For this review, take the finished solid that the model builds, in its own axes (mm). A direction names the side the tool comes from. Round coordinates to 2 decimals unless told otherwise and drop trailing zeros. Order: outer loops, then holes, each group sorted by start corner. A loop starts at its lowest first (then second) coordinate and runs counter-clockwise, first axis right, second up. Notation, with made-up numbers: (18.5, -3) - (37.5, -3) arc R12 ccw to (37.5, 5) - close; hole circle Ø7 at (1.25, 83). An arc over 180 degrees is marked (long way). One line per item, written item: value.
```python
from build123d import *

# Parameters (mm, degrees)
SKETCH1_W           = 10
SKETCH1_H           = 290
SKETCH2_R           = 15
BOSS_EXTRUDE1_DEPTH = 50


with BuildPart() as part:
    # Sketch1 → Revolve1 (revolve)
    with BuildSketch(Plane.XY, mode=Mode.PRIVATE) as revolve1_sk:
        with Locations((-5, 0)):
            Rectangle(SKETCH1_W, SKETCH1_H)
    revolve(revolve1_sk.sketch.rotate(Axis((0, 145, 0), (0, -1, 0)), 270), axis=Axis((0, 145, 0), (0, -1, 0)))

    # Sketch2 → Boss-Extrude1 (add, symmetric)
    with BuildSketch(Plane(origin=(0, 0, 0), x_dir=(0, 0, -1), z_dir=(1, 0, 0))):
        with Locations((0, 145)):
            Circle(SKETCH2_R)
    boss_extrude1 = extrude(amount=BOSS_EXTRUDE1_DEPTH, both=True)

    # Mirror1: Boss-Extrude1 across plane
    add(boss_extrude1.mirror(Plane.ZX))


solid = part.part
```
Item 1: Take a section at A-A (z = 0). Write out the cut boundary in (x, y), plus the area to 3 significant figures.
Returned:
outline: (-50, -160) - (50, -160) - (50, -130) - (10, -130) - (10, 130) - (50, 130) - (50, 160) - (-50, 160) - (-50, 130) - (-10, 130) - (-10, -130) - (-50, -130) - close
area: 11,200 mm^2
Item 2: Machinability: for faces 1 (the flat face through (-50, 145, 0)), 2 (the cylindrical face through (9.76, 1.87, -2.17)), which of the approach directions +Z, -Z, +X, -X, +Y, -Y give a long, thin tool a straight path to every point of the face, cutting with its end or side? Answer none if there is none.
Returned:
face 1: +Z, -Z, -X, +Y, -Y
face 2: none
Item 3: Take a section at C-C (y = -49). Write out the cut boundary in (x, z).
Returned:
outline: circle Ø20 at (0, 0)
Item 4: For P1, Ø3, axis at y = 120, z = 6, coming from the -X side; P2, Ø8, axis at y = -62, z = 10.5, coming from the +X side; P3, Ø6, axis at x = 30.5, z = 7.5, coming from the +Y side, all flat-tipped, find the tip position at first contact; note any pin that passes through.
Returned:
P1: x = -8.93
P2: x = 7.6
P3: y = 159.31
Item 5: Wall thickness on line 1 (Y direction, x = -34.5, z = -12); line 2 (Y direction, x = -23.5, z = -10); line 3 (Y direction, x = -5, z = 1): over which ranges is each line inside the solid? List them lowest first.
Returned:
line 1: -154 to -136, 136 to 154
line 2: -156.18 to -133.82, 133.82 to 156.18
line 3: -159.97 to 159.97
Item 6: Take a section at D-D (x = 0). Write out the cut boundary in (y, z).
Returned:
outline: (-133.82, -10) - (133.82, -10) arc R15 ccw (long way) to (133.82, 10) - (-133.82, 10) arc R15 ccw (long way) to start
Item 7: Take a section at B-B (x = -16.5). Write out the cut boundary in (y, z), plus the area to 3 significant figures.
Returned:
outline: circle Ø30 at (-145, 0); circle Ø30 at (145, 0)
area: 1,410 mm^2
Item 8: The part is to be moulded in two halves that separate along Y. For faces 3 (the cylindrical face through (0.7, -159.872, 1.953)), 4 (the flat face through (50, 145, 0)), say which applies: +Y half, -Y half, draft (parallel to the pull), parting line (faces both ways), or undercut.
Returned:
face 3: undercut
face 4: draft
